Here's how the part is built. I have some questions about the finished solid (model axes, mm). A direction names the side the tool comes from. Coordinates: 2 decimals unless noted, no trailing zeros. Write each loop counter-clockwise with the first axis right and the second up, starting at its lowest first coordinate (ties: lowest second). Pieces come first, ordered by that corner, then holes.
```python
from build123d import *

# Parameters (mm, degrees)
SKETCH3_W                       = 23
SKETCH3_H                       = 8
EXTRUDE1_DEPTH                  = 100
M5_TAPPED_HOLE1_D               = 4.2
M4_TAPPED_HOLE1_D               = 3.3
M4_TAPPED_HOLE1_DEPTH           = 10
M4_TAPPED_HOLE1_TIP             = 0.991420021
M4_TAPPED_HOLE1_ON_FACE_2_D     = 3.3
M4_TAPPED_HOLE1_ON_FACE_2_DEPTH = 10
M4_TAPPED_HOLE1_ON_FACE_2_TIP   = 0.991420021
M3_TAPPED_HOLE1_REACH           = 25
M3_TAPPED_HOLE1_BORE_R          = 1.25


with BuildPart() as part:
    # Sketch3 → Extrude1 (new body)
    with BuildSketch(Plane.XY):
        with Locations((11.5, 4)):
            Rectangle(SKETCH3_W, SKETCH3_H)
    extrude(amount=EXTRUDE1_DEPTH)

    # M5 Tapped Hole1 (through all)
    with Locations(Plane(origin=(11.5, 8, 90), x_dir=(0, 0, 1), z_dir=(0, 1, 0))):
        with Locations((0, 0), (-80, 0)):
            Hole(M5_TAPPED_HOLE1_D / 2)

    # M4 Tapped Hole1
    with Locations(Plane(origin=(6, 4, 100), x_dir=(1, 0, 0), z_dir=(0, 0, 1))):
        with Locations((0, 0), (13, 0)):
            Hole(M4_TAPPED_HOLE1_D / 2, depth=M4_TAPPED_HOLE1_DEPTH)
            with Locations((0, 0, -(M4_TAPPED_HOLE1_DEPTH + M4_TAPPED_HOLE1_TIP / 2))):  # 118° drill point
                Cone(0, M4_TAPPED_HOLE1_D / 2, M4_TAPPED_HOLE1_TIP, mode=Mode.SUBTRACT)

    # M4 Tapped Hole1 on face 2
    with Locations(Plane(origin=(19, 4, 0), x_dir=(-1, 0, 0), z_dir=(0, 0, -1))):
        with Locations((0, 0), (15, 0)):
            Hole(M4_TAPPED_HOLE1_ON_FACE_2_D / 2, depth=M4_TAPPED_HOLE1_ON_FACE_2_DEPTH)
            with Locations((0, 0, -(M4_TAPPED_HOLE1_ON_FACE_2_DEPTH + M4_TAPPED_HOLE1_ON_FACE_2_TIP / 2))):  # 118° drill point
                Cone(0, M4_TAPPED_HOLE1_ON_FACE_2_D / 2, M4_TAPPED_HOLE1_ON_FACE_2_TIP, mode=Mode.SUBTRACT)

    # M3 Tapped Hole1 bore (on position points) → M3 Tapped Hole1 (cut, up to next)
    with BuildSketch(Plane(origin=(0, 4, 4), x_dir=(0, 0, -1), z_dir=(-1, 0, 0)), mode=Mode.PRIVATE) as m3_tapped_hole1_sk1:
        Circle(M3_TAPPED_HOLE1_BORE_R)
    m3_tapped_hole1_tool1 = extrude(m3_tapped_hole1_sk1.sketch, amount=-M3_TAPPED_HOLE1_REACH, mode=Mode.PRIVATE) & part.part
    add(m3_tapped_hole1_tool1.solids().sort_by_distance((0, 4, 4))[0], mode=Mode.SUBTRACT)


solid = part.part
```
1) We'd pull the mould along X, two halves only. Please class faces 1 (the face through (1.441, 5.109, 3.423)), 2 (the face through (7.65, 4.07, 94.93)), 3 (the face through (0, 4, 49)), 4 (the face through (6.1, 3.7, 89.2)): pulls with the +X half, pulls with the -X half, needs draft (parallel to the pull), parting line crosses it, or undercut.
Values follow:
face 1: needs draft
face 2: undercut
face 3: pulls with the -X half
face 4: undercut
2) On a 3-axis mill with a long thin cutter (end or side, diameter ignored), from which of +Z, -Z, +X, -X, +Y, -Y can I reach the whole of each face in a straight line? I mean faces 5 (the face through (20.31, 3, 94.93)), 6 (the face through (11.59, 3.94, 12.1)), 7 (the face through (17.69, 3, 5.07)). Say none if no direction works.
Values follow:
face 5: +Z
face 6: +Y, -Y
face 7: -Z
3) Imagine slicing it at A-A on x = 11.5. Please give me the cut outline in (y, z), then the cut area to 3 significant figures.
Values follow:
outline: (0, 0) - (8, 0) - (8, 7.9) - (0, 7.9) - close; (0, 12.1) - (8, 12.1) - (8, 87.9) - (0, 87.9) - close; (0, 92.1) - (8, 92.1) - (8, 100) - (0, 100) - close
area: 733 mm2
4) Imagine slicing it at B-B on z = 4. Please give me the cut outline in (x, y), then the cut area to 3 significant figures.
Values follow:
outline: (0, 0) - (23, 0) - (23, 8) - (0, 8) - (0, 5.25) - (2.92, 5.25) arc R1.65 cw (long way) to (2.92, 2.75) - (0, 2.75) - close; hole circle Ø3.3 at (19, 4)
area: 161 mm2
5) I need wall thicknesses on probe 1 along X at (y, z) = (4, 6); probe 2 along X at (y, z) = (4, 96.5); probe 3 along Z at (x, y) = (10.75, 2.75). Which ranges of each line are inside material? Lowest first, please.
Values follow:
probe 1: x = 0 to 2.35, 5.65 to 17.35, 20.65 to 23
probe 2: x = 0 to 4.35, 7.65 to 17.35, 20.65 to 23
probe 3: z = 0 to 8.04, 11.96 to 88.04, 91.96 to 100
6) Will these pins go through, and if not, where does the flat tip stop? pin 1 (3.5 mm diameter, centred on x = 11.5, z = 10, fed in from -Y); pin 2 (2.5 mm diameter, centred on x = 19, y = 4, fed in from +Z); pin 3 (2 mm diameter, centred on y = 4, z = 4, fed in from -X).
Values follow:
pin 1: passes through
pin 2: stops at z = 89.76
pin 3: stops at x = 5.31
